Part model, mm, in its own coordinate system. A direction names the side the tool comes from. Round coordinates to 2 decimals unless told otherwise and drop trailing zeros. Loops run counter-clockwise (first coordinate to the right, second up) from the corner with the lowest first, then second, coordinate; pieces in that order, holes last. Notation, with made-up numbers: M 77,-10.75 L 117,-10.75 A15 cw 117,-5.75 Z; hole C -33.5,-13 d2. An arc over 180 degrees is marked long. Put each result on its own line as item: value. Start each with the question number.
```python
from build123d import *

# Parameters (mm, degrees)
SKETCH_1_R      = 3.5
SKETCH_1_R_2    = 2.5
EXTRUDE_1_DEPTH = 5


with BuildPart() as part:
    # Эскиз1 → Бобышка-Вытянуть1 (new body)
    with BuildSketch(Plane.XY):
        with BuildLine():
            Line((-17.142857316, -25), (17.142857316, -25))
            ThreePointArc((17.142857316, -25), (19.996912391, -25.894592635), (21.829680805, -28.258252147))
            ThreePointArc((21.829680805, -28.258252147), (30.0520382, -30.0520382), (28.258252147, -21.829680805))
            ThreePointArc((28.258252147, -21.829680805), (25.894592635, -19.996912391), (25, -17.142857316))
            Line((25, -17.142857316), (25, 17.142857316))
            ThreePointArc((25, 17.142857316), (25.894592635, 19.996912391), (28.258252147, 21.829680805))
            ThreePointArc((28.258252147, 21.829680805), (30.0520382, 30.0520382), (21.829680805, 28.258252147))
            ThreePointArc((21.829680805, 28.258252147), (19.996912391, 25.894592635), (17.142857316, 25))
            Line((17.142857316, 25), (-17.142857316, 25))
            ThreePointArc((-17.142857316, 25), (-19.996912391, 25.894592635), (-21.829680805, 28.258252147))
            ThreePointArc((-21.829680805, 28.258252147), (-30.0520382, 30.0520382), (-28.258252147, 21.829680805))
            ThreePointArc((-28.258252147, 21.829680805), (-25.894592635, 19.996912391), (-25, 17.142857316))
            Line((-25, 17.142857316), (-25, -17.142857316))
            ThreePointArc((-25, -17.142857316), (-25.894592635, -19.996912391), (-28.258252147, -21.829680805))
            ThreePointArc((-28.258252147, -21.829680805), (-30.0520382, -30.0520382), (-21.829680805, -28.258252147))
            ThreePointArc((-21.829680805, -28.258252147), (-19.996912391, -25.894592635), (-17.142857316, -25))
        make_face()
        Circle(SKETCH_1_R, mode=Mode.SUBTRACT)
        with Locations((-26.516504294, 26.516504295)):
            Circle(SKETCH_1_R_2, mode=Mode.SUBTRACT)
        with Locations((26.516504295, 26.516504294)):
            Circle(SKETCH_1_R_2, mode=Mode.SUBTRACT)
        with Locations((26.516504294, -26.516504295)):
            Circle(SKETCH_1_R_2, mode=Mode.SUBTRACT)
        with Locations((-26.516504295, -26.516504294)):
            Circle(SKETCH_1_R_2, mode=Mode.SUBTRACT)
    extrude(amount=EXTRUDE_1_DEPTH)


solid = part.part
```
1. Wall check: L1, parallel to Y at x = 0, z = 1.2; L2, parallel to X at y = 8, z = 3.35. Give the ranges that are in metal, low to high.
2. Mould opens along X. For faces 4 (the flat face through (25, 0, 2)), 5 (the flat face through (0, 7, 5)), 6 (the cylindrical face through (24.02, -26.41, 2.46)) say: released by +X, released by -X, zero draft, split by the parting line, or undercut.
3. Cut at D-D, the plane y = 10. Give the cut face in (x, z).
4. Cut at C-C, the plane z = 0.85. Give the cut face in (x, y), and give its area (3 significant figures).
5. Cut at A-A, the plane x = 0. Give the cut face in (y, z), and give its area (3 significant figures).
6. Which spindle directions (+Z, -Z, +X, -X, +Y, -Y) get a long thin tool onto all of the face, cutting with end or side? Do faces 1 (the flat face through (0, -25, 2)), 2 (the flat face through (-25, 0, 2)), 3 (the flat face through (0, 25, 2)). Say none if no direction does.
7. Drop flat-ended pins along their axis: pin 1 (3 mm diameter, centred on y = -21.5, z = 3.5, fed in from +X); pin 2 (4.5 mm diameter, centred on x = 26.52, y = 26.52, fed in from -Z); pin 3 (2.5 mm diameter, centred on y = -6, z = 1.5, fed in from -X); pin 4 (2 mm diameter, centred on x = -11, z = 1.5, fed in from -Y). Give the stop position or say it passes through.
Results list:
1. L1: y = -25 to -3.5, 3.5 to 25
1. L2: x = -25 to 25
2. face 4: released by +X
2. face 5: zero draft
2. face 6: undercut
3. outline: M -25,0 L 25,0 L 25,5 L -25,5 Z
4. outline: M -28.26,-21.83 A5 ccw long -21.83,-28.26 A5 cw -17.14,-25 L 17.14,-25 A5 cw 21.83,-28.26 A5 ccw long 28.26,-21.83 A5 cw 25,-17.14 L 25,17.14 A5 cw 28.26,21.83 A5 ccw long 21.83,28.26 A5 cw 17.14,25 L -17.14,25 A5 cw -21.83,28.26 A5 ccw long -28.26,21.83 A5 cw -25,17.14 L -25,-17.14 A5 cw Z; hole C -26.52,-26.52 d5; hole C -26.52,26.52 d5; hole C 0,0 d7; hole C 26.52,-26.52 d5; hole C 26.52,26.52 d5
4. area: 2,700 mm^2
5. outline: M -25,0 L -3.5,0 L -3.5,5 L -25,5 Z; M 3.5,0 L 25,0 L 25,5 L 3.5,5 Z
5. area: 215 mm^2
6. face 1: +Z, -Z, -Y
6. face 2: +Z, -Z, -X
6. face 3: +Z, -Z, +Y
7. pin 1: stops at x = 30.07
7. pin 2: passes through
7. pin 3: stops at x = -25
7. pin 4: stops at y = -25
